The listing builds one solid part. Answer for the finished solid, in the listing's coordinates (mm). A direction names the side the tool comes from. Coordinates: 2 decimals unless noted, no trailing zeros. Loops run counter-clockwise (first coordinate to the right, second up) from the corner with the lowest first, then second, coordinate; pieces in that order, holes last. Notation, with made-up numbers: (29.5, -15.75) - (44.5, -15.75) arc R8 ccw to (44.5, -2.75) - close; hole circle Ø1 at (-24.75, 56). An arc over 180 degrees is marked (long way). Write each question's results on one line, items separated by ' | '. Start each with the question number.
(1) Find section C-C on x = 1. Determine the outline of the cut face in (y, z).
(2) Find section B-B on z = 462. Determine the outline of the cut face in (x, y).
(3) Find section A-A on y = -1.5. Determine the outline of the cut face in (x, z).
(4) Consider line 1 (X direction, y = -2.5, z = 191); line 2 (Y direction, x = 4, z = 481). Determine where each line is inside the solid, lowest interval first. Write a range as from..to.
(5) For faces 1 (the flat face through (-24.434, 0, 345)), 2 (the flat face through (-8, -10.7, 345)), determine the directions among +Z, -Z, +X, -X, +Y, -Y from which every point of the face is accessible in a straight line to the end or side of a thin tool.
(6) Given pin 1 Ø1 at (x, z) = (3.5, 431) entering from +Y, flat-ended and moving along its own axis, determine where the tip first touches the part or whether it passes through.
Autodesk Inventor part; units mm, degrees
ref_plane "YZ Plane" through (0, 0, 0) normal (1, 0, 0) x (0, 1, 0)
ref_plane "XZ Plane" through (0, 0, 0) normal (0, 1, 0) x (-1, 0, 0)
ref_plane "XY Plane" through (0, 0, 0) normal (0, 0, 1) x (1, 0, 0)
sketch "Skizze1" plane through (0, 0, 0) normal (0, 0, 1) x (1, 0, 0)
  line L0 (-25.9341, 8.8004) -> (-25.9341, -10.6996)
  line L1 (-25.9341, -10.6996) -> (9.5659, -10.6996)
  line L2 (9.5659, -10.6996) -> (9.5659, 8.8004)
  line L3 (9.5659, 8.8004) -> (8.0659, 8.8004)
  line L4 (8.0659, 8.8004) -> (8.0659, -9.1996)
  line L5 (8.0659, -9.1996) -> (-24.4341, -9.1996)
  line L6 (-24.4341, -9.1996) -> (-24.4341, 8.8004)
  line L7 (-24.4341, 8.8004) -> (-25.9341, 8.8004)
  point P0 (0, 0)
  dimension "d0" = 35.5
  dimension "d1" = 32.5
  dimension "d2" = 1.5
  dimension "d3" = 19.5
  dimension "d4" = 1.5
extrude "Extrusion1" add sketch "Skizze1" along normal blind 700
properties part number "Grundstange Bauhaus"
Values:
1) outline: (-10.7, 0) - (-9.2, 0) - (-9.2, 700) - (-10.7, 700) - close
2) outline: (-25.93, -10.7) - (9.57, -10.7) - (9.57, 8.8) - (8.07, 8.8) - (8.07, -9.2) - (-24.43, -9.2) - (-24.43, 8.8) - (-25.93, 8.8) - close
3) outline: (-25.93, 0) - (-24.43, 0) - (-24.43, 700) - (-25.93, 700) - close; (8.07, 0) - (9.57, 0) - (9.57, 700) - (8.07, 700) - close
4) line 1: x = -25.93..-24.43, 8.07..9.57 | line 2: y = -10.7..-9.2
5) face 1: +Z, -Z, +Y | face 2: +Z, -Z, +X, -X, -Y
6) pin 1: stops at y = -9.2
